Geometry check sheet. Reference: the model listing, model coordinates, mm. Face numbers are marked on the shaded views. A direction names the side the tool comes from. Round coordinates to 2 decimals unless told otherwise and drop trailing zeros. Write each loop counter-clockwise with the first axis right and the second up, starting at its lowest first coordinate (ties: lowest second). Pieces come first, ordered by that corner, then holes. Notation, with made-up numbers: M -11,-1.5 L -2,-1.5 A24 ccw -2,37.5 Z; hole C 31.5,21.5 d4. An arc over 180 degrees is marked long. Put each result on its own line as item: value. Start each with the question number.
(1) Gauge pin test, flat ends, axial feed: pin 1 (3 mm diameter, centred on y = -13.5, z = -4.5, fed in from +X); pin 2 (3 mm diameter, centred on x = 51.5, y = 4.5, fed in from +Z); pin 3 (10 mm diameter, centred on x = 32, z = 2.5, fed in from +Y). Record the tip position at first contact, or that the pin passes through.
(2) Section check A-A on x = 79.5. Record the cut outline in (y, z), then the cut area to 3 significant figures.
(3) Tool access check on the marked faces 1 and 2. Record the directions out of +Z, -Z, +X, -X, +Y, -Y that give a thin tool (end or side, any length) a straight path to the whole face; none if there is none.
(4) Material ranges on probe 1 along X at (y, z) = (14.5, 0.5); probe 2 along Y at (x, z) = (60, 0); probe 3 along Y at (x, z) = (98.5, 5), recorded low to high.
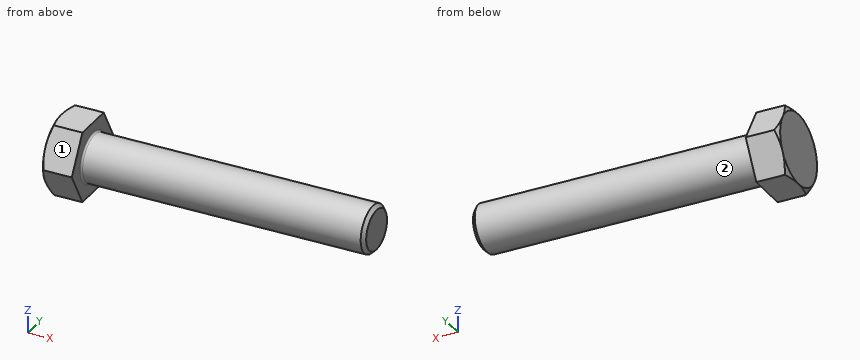
Autodesk Inventor part; units mm, degrees
ref_plane "Work Plane1" through (1.525, 0, 0) normal (0, 0, 1) x (1, 0, 0)
ref_plane "YZ Plane" through (0, 0, 0) normal (1, 0, 0) x (0, 1, 0)
ref_plane "XZ Plane" through (0, 0, 0) normal (0, 1, 0) x (-1, 0, 0)
sketch "Sketch1" plane through (0, 0, 0) normal (0, 0, 1) x (1, 0, 0)
  line L0 (0, 10) -> (120, 10)
  line L1 (120, 10) -> (120, 0)
  line L2 (120, 0) -> (0, 0)
  line L3 (-24, 0) -> (144, 0)
  line L4 (0, -2) -> (0, 12)
  line L5 (0, 10) -> (0, 0)
  dimension "d2" = 20
  dimension "d59" = 120
revolve "Body" add sketch "Sketch1" angle 360 about axis through (120, 0, 0) along (-1, 0, 0)
sketch "Sketch2" plane through (0, 0, 0) normal (-1, 0, 0) x (0, 0, 1)
  line L0 (0, 17.3205) -> (15, 8.6603)
  line L1 (15, 8.6603) -> (15, -8.6603)
  line L2 (15, -8.6603) -> (0, -17.3205)
  line L3 (0, -17.3205) -> (-15, -8.6603)
  line L4 (-15, -8.6603) -> (-15, 8.6603)
  line L5 (-15, 8.6603) -> (0, 17.3205)
  line L6 (-21, 0) -> (21, 0)
  line L7 (0, 24.2487) -> (0, -24.2487)
  point P0 (0, 0)
  point P1 (0, 0)
  dimension "d11" = 30
extrude "Head" add sketch "Sketch2" along normal blind 13.4
sketch "Sketch4" plane through (0, 0, 0) normal (0, 0, 1) x (1, 0, 0)
  line L0 (-11.6679, 18) -> (-13.4, 15)
  line L1 (-1.1, 0) -> (-0.234, 0)
  line L2 (-16.0332, 0) -> (2.3992, 0)
  line L3 (-13.4, 18) -> (-11.6679, 18)
  line L4 (-13.4, 15) -> (-13.4, 18)
  line L5 (0, 21.6) -> (0, -3.6)
  dimension "d65" = 30
  dimension "d67" = 30
  dimension "d68" = 36
  dimension "d69" = 13.4
revolve "Chamfer1" cut sketch "Sketch4" angle 360 about axis through (-1.1, 0, 0) along (1, 0, 0)
thread "Thread"
chamfer "Chamfer2" distance 1.5336 distance2 1.5337 1 edges at (120, -10, 0) measured on face at (120, -2.6738, -2.9356)
fillet "Fillet" radius 0.8 1 edges at (0, -10, 0)
ref_plane "Work Plane1" through (1.525, 0, 0) normal (0, 0, 1) x (1, 0, 0)
equation "\"d2\" = GD"
equation "\"d59\" = NLG"
equation "\"d11\" = SW"
equation "\"d3\" = KOH"
equation "\"d15\" = GEL"
equation "\"d6\" = -0.5 * SPD + 0.5 * GD"
equation "\"d71\" = RR1"
equation "\"d65\" = SW"
equation "\"d67\" = ANG1"
equation "\"d68\" = 1.2 * SW"
equation "\"d69\" = KOH"
equation "\"NLG\" = 120"
equation "\"GD\" = NND"
equation "\"KOH\" = 13.4"
equation "\"GEL\" = 46"
equation "\"SW\" = 30"
equation "\"SPD\" = NND - 1.2269 * PTC"
equation "\"SD\" = 0"
equation "\"ANG1\" = 30deg"
equation "\"GAL\" = 0.61345 * PTC"
equation "\"GUL\" = 0.61345 * PTC"
equation "\"RR\" = 0.1"
equation "\"RR1\" = 0.8"
equation "\"GD1\" = THREADDIA - 1.2269 * PTC"
equation "\"TOA\" = 30deg"
equation "\"PTC\" = 2.5"
equation "\"KOH1\" = 8.8"
equation "\"E0\" = 1.155 * SW"
properties part number "ANSI B18.2.3.5M - M20 x 2,5 x 120" material "Steel, Mild"
Answers follow:
1. pin 1: stops at x = 0
1. pin 2: stops at z = 9.54
1. pin 3: stops at y = 10
2. outline: C 0,0 d20
2. area: 314 mm^2
3. face 1: +Z, +X, -X, -Y
3. face 2: +X
4. probe 1: x = -13.4 to 0
4. probe 2: y = -10 to 10
4. probe 3: y = -8.66 to 8.66
